The model under review builds one solid part; all positions refer to its coordinate system, in mm. Face numbers are marked on the shaded views. A direction names the side the tool comes from. Coordinates: 2 decimals unless noted, no trailing zeros. Order: outer loops, then holes, each group sorted by start corner. A loop starts at its lowest first (then second) coordinate and runs counter-clockwise, first axis right, second up. Notation, with made-up numbers: (-13.75, 50.25) -> (40.25, 50.25) arc R27 ccw to (40.25, 79.25) -> close; hole circle Ø10 at (24.25, 13.5). An arc over 180 degrees is marked (long way). Put each result on its own line as item: value.
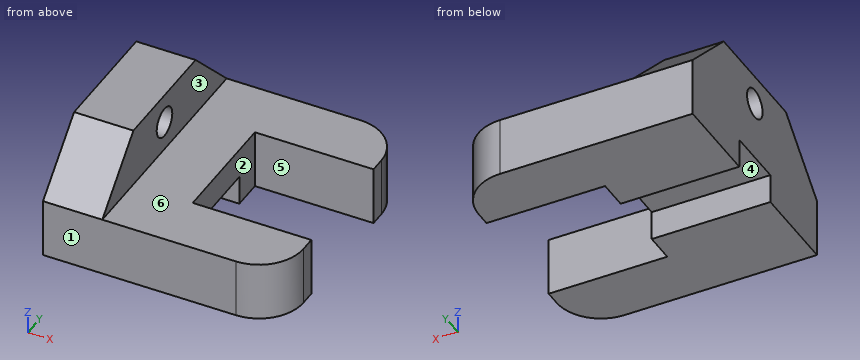
from build123d import *

# Parameters (mm, degrees)
F1_DEPTH = 50.8
F3_DEPTH = 50.8
F4_R     = 12.7
F5_DEPTH = 50.8
F6_W     = 50.8
F6_H     = 25.4
F7_DEPTH = 101.6


with BuildPart() as f1:
    # F0 (on Top) → F1 (new body)
    with BuildSketch(Plane.XY):
        with BuildLine():
            Line((165.1, 203.2), (0, 203.2))
            Line((0, 203.2), (0, 0))
            Line((0, 0), (165.1, 0))
            ThreePointArc((165.1, 0), (192.040768, 11.159232), (203.2, 38.1))
            Line((203.2, 38.1), (203.2, 50.8))
            Line((203.2, 50.8), (101.6, 50.8))
            Line((101.6, 50.8), (101.6, 152.4))
            Line((101.6, 152.4), (203.2, 152.4))
            Line((203.2, 152.4), (203.2, 165.1))
            ThreePointArc((203.2, 165.1), (192.040768, 192.040768), (165.1, 203.2))
        make_face()
    extrude(amount=F1_DEPTH)

    # F2 (on Right) → F3 (join)
    with BuildSketch(Plane.YZ):
        Polygon((152.4, 101.6), (50.8, 101.6), (0, 50.8), (203.2, 50.8), align=None)
    extrude(amount=F3_DEPTH)

    # F4 (on face) → F5 (cut)
    with BuildSketch(Plane.YZ.offset(50.8)):
        with Locations((101.6, 76.2)):
            Circle(F4_R)
    extrude(amount=-F5_DEPTH, mode=Mode.SUBTRACT)

    # F6 (on face) → F7 (cut)
    with BuildSketch(Plane.YZ.offset(101.6)):
        with Locations((101.6, 12.7)):
            Rectangle(F6_W, F6_H)
    extrude(amount=-F7_DEPTH, mode=Mode.SUBTRACT)


solid = f1.part
Item 1: Consider section D-D on z = 39.5. Write out the cut boundary in (x, y), and give its area (3 significant figures).
Answers below:
outline: (0, 0) -> (165.1, 0) arc R38.1 ccw to (203.2, 38.1) -> (203.2, 50.8) -> (101.6, 50.8) -> (101.6, 152.4) -> (203.2, 152.4) -> (203.2, 165.1) arc R38.1 ccw to (165.1, 203.2) -> (0, 203.2) -> close
area: 30,300 mm^2
Item 2: For pin 1 Ø12 at (y, z) = (110, 90.5) entering from +X; pin 2 Ø15 at (y, z) = (102.5, 28.5) entering from +X, all flat-tipped, find the tip position at first contact; note any pin that passes through.
Answers below:
pin 1: x = 50.8
pin 2: x = 101.6
Item 3: For line 1 (Z direction, x = 24.5, y = 101.6); line 2 (Y direction, x = 56.5, z = 23.5); line 3 (Z direction, x = 82.5, y = 11), list the stretches that pass through material, from the lowest coordinate up. Write a range as from..to.
Answers below:
line 1: 25.4..63.5, 88.9..101.6
line 2: 0..76.2, 127..203.2
line 3: 0..50.8
Item 4: For the marked faces 4, 5 and 6, list the 3-axis set-ups (+Z, -Z, +X, -X, +Y, -Y) from which the entire face can be reached by the end or side of a thin tool; tool diameter is ignored.
Answers below:
face 4: -Z, +X, -X
face 5: +Z, -Z, +X
face 6: +Z, +X, +Y, -Y
Item 5: Consider section B-B on z = 76.2. Write out the cut boundary in (x, y), and give its area (3 significant figures).
Answers below:
outline: (0, 25.4) -> (50.8, 25.4) -> (50.8, 88.9) -> (0, 88.9) -> close; (0, 114.3) -> (50.8, 114.3) -> (50.8, 177.8) -> (0, 177.8) -> close
area: 6,450 mm^2
Item 6: Consider section C-C on x = 67. Write out the cut boundary in (y, z).
Answers below:
outline: (0, 0) -> (76.2, 0) -> (76.2, 25.4) -> (127, 25.4) -> (127, 0) -> (203.2, 0) -> (203.2, 50.8) -> (0, 50.8) -> close
Item 7: Consider section A-A on y = 101.6. Write out the cut boundary in (x, z), and give its area (3 significant figures).
Answers below:
outline: (0, 25.4) -> (101.6, 25.4) -> (101.6, 50.8) -> (50.8, 50.8) -> (50.8, 63.5) -> (0, 63.5) -> close; (0, 88.9) -> (50.8, 88.9) -> (50.8, 101.6) -> (0, 101.6) -> close
area: 3,870 mm^2
Item 8: Mouldability with a two-part tool opening along Y and no side actions: class the marked faces 1, 2 and 3 as +Y half, -Y half, draft (parallel to the pull), parting line (faces both ways), or undercut.
Answers below:
face 1: -Y half
face 2: undercut
face 3: draft
